Input: part model. Units: mm. Frame: model coordinates. Face numbers are marked on the shaded views. Coordinates: 2 decimals unless noted, no trailing zeros. Loops run counter-clockwise (first coordinate to the right, second up) from the corner with the lowest first, then second, coordinate; pieces in that order, holes last. Notation, with made-up numbers: (80, 11.5) - (101, 11.5) arc R9 ccw to (101, 22.5) - close; hole circle Ø9 at (31.5, 27). An arc over 180 degrees is marked (long way). Write item = value, one per line. Start each with the question number.
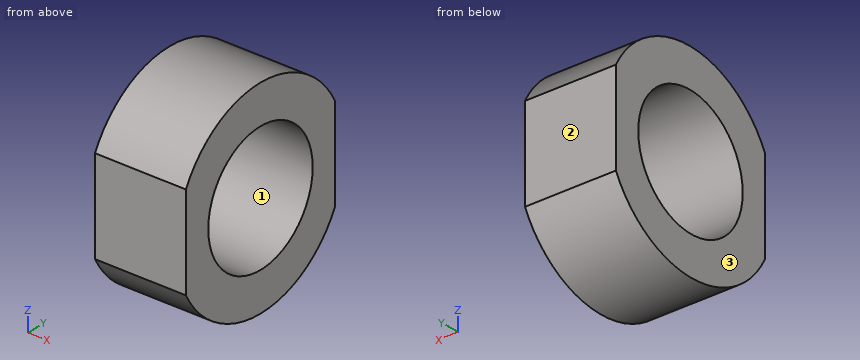
from build123d import *

# Parameters (mm, degrees)
F0_R     = 14
F1_DEPTH = 20


with BuildPart() as f1:
    # F0 (on Right) → F1 (new body)
    with BuildSketch(Plane.YZ):
        with BuildLine():
            Line((-20, 10.307764), (-20, -10.307764))
            ThreePointArc((-20, -10.307764), (0, -22.5), (20, -10.307764))
            Line((20, -10.307764), (20, 10.307764))
            ThreePointArc((20, 10.307764), (0, 22.5), (-20, 10.307764))
        make_face()
        Circle(F0_R, mode=Mode.SUBTRACT)
    extrude(amount=F1_DEPTH)


solid = f1.part
Item 1: Pull-direction query (Y, two-part tool) for the marked faces 1, 2 and 3; classes: pulls with the +Y half, pulls with the -Y half, needs draft (parallel to the pull), parting line crosses it, or undercut.
Item 2: Pin query (flat end, axial travel): pin 1 (4 mm diameter, centred on x = 2.5, y = -14, fed in from +Z); pin 2 (10 mm diameter, centred on x = 6.5, y = 12, fed in from -Z); pin 3 (6 mm diameter, centred on x = 10, y = 7.5, fed in from -Z); pin 4 (6 mm diameter, centred on y = 6, z = 8, fed in from -X). Return the tip coordinate at first contact, or that it passes through.
Item 3: Cut plane B-B on z = 0. Return loops of the section in (x, y).
Item 4: Cut plane C-C on x = 12. Return loops of the section in (y, z), plus the area to 3 significant figures.
Item 5: Cut plane D-D on z = -19. Return loops of the section in (x, y), plus the area to 3 significant figures.
Item 6: Ray query, line 1 (Z direction, x = 7.5, y = 0); line 2 (Y direction, x = 16.25, z = 6); line 3 (Y direction, x = 10.5, z = -7). Return the intervals inside material, ascending.
Item 7: Cut plane A-A on y = 0. Return loops of the section in (x, z).
Recorded:
q1.face_1 = undercut
q1.face_2 = pulls with the +Y half
q1.face_3 = needs draft
q2.pin_1 = 19.03
q2.pin_2 = -21.38
q2.pin_3 = -22.05
q2.pin_4 = through
q3.outline = (0, -20) - (20, -20) - (20, -14) - (0, -14) - close; (0, 14) - (20, 14) - (20, 20) - (0, 20) - close
q4.outline = (-20, -10.31) arc R22.5 ccw to (20, -10.31) - (20, 10.31) arc R22.5 ccw to (-20, 10.31) - close; hole circle Ø28 at (0, 0)
q4.area = 905 mm²
q5.outline = (0, -12.05) - (20, -12.05) - (20, 12.05) - (0, 12.05) - close
q5.area = 482 mm²
q6.line_1 = -22.5 to -14, 14 to 22.5
q6.line_2 = -20 to -12.65, 12.65 to 20
q6.line_3 = -20 to -12.12, 12.12 to 20
q7.outline = (0, -22.5) - (20, -22.5) - (20, -14) - (0, -14) - close; (0, 14) - (20, 14) - (20, 22.5) - (0, 22.5) - close
